Part model, mm, in its own coordinate system. A direction names the side the tool comes from. Coordinates: 2 decimals unless noted, no trailing zeros. Loops run counter-clockwise (first coordinate to the right, second up) from the corner with the lowest first, then second, coordinate; pieces in that order, holes last. Notation, with made-up numbers: (15, 34.25) - (60, 34.25) arc R35 ccw to (60, 73.25) - close; hole circle Ø5 at (41, -24). An arc over 180 degrees is marked (long way). Use a Markdown table: item, result. Add a question column.
1) Tool access for faces 4 (the face through (4.38, -8.43, 52.48)), 5 (the face through (-2.38, -10.74, 13.74)), 6 (the face through (8.11, 2.55, 139.47)), 7 (the face through (-7, 0, 122)): list every direction of +Z, -Z, +X, -X, +Y, -Y with a clear straight run to the whole face (end or side of a thin tool).
2) Probe probe 1 along Y at (x, z) = (0, 158); probe 2 along Z at (x, y) = (5, -5.5); probe 3 along Z at (x, y) = (-7.5, -4.5). List the from-to ranges inside material, lowest first. Write a range as [from, to].
3) Pull direction Z, two halves, no side cores. Call faces 1 (the face through (4.57, 7.167, 5.676)), 2 (the face through (-7, 0, 142)), 3 (the face through (2, -2, 0)): +Z half, -Z half, draft (parallel to the pull), parting line (faces both ways), or undercut.
4) Drop flat-ended pins along their axis: P1, Ø10, axis at x = 9, z = 120, coming from the +Y side; P2, Ø4, axis at x = 9.5, y = -2.5, coming from the -Z side; P3, Ø5, axis at y = -4.5, z = 23.5, coming from the -X side; P4, Ø8, axis at y = 11.5, z = 121.5, coming from the -X side. Give the stop position or say it passes through.
5) Band-saw the part on A-A (z = 104). Give the cut face in (x, y), plus the area to 3 significant figures.
from build123d import *

# Parameters (mm, degrees)
SKETCH1_R       = 8.5
EXTRUDE1_DEPTH  = 11
SKETCH2_R       = 6.5
EXTRUDE2_DEPTH  = 2
SKETCH3_R       = 11
EXTRUDE3_DEPTH  = 3
SKETCH4_R       = 9.5
EXTRUDE4_DEPTH  = 80
SKETCH5_R       = 11
EXTRUDE5_DEPTH  = 23
SKETCH6_R       = 8.25
EXTRUDE6_DEPTH  = 1
SKETCH7_R       = 8.5
EXTRUDE7_DEPTH  = 40
CHAMFER1_SIZE   = 0.5
CHAMFER2_SIZE   = 1.5
SKETCH8_R       = 2
EXTRUDE8_DEPTH  = 6
CHAMFER3_SIZE   = 2
EXTRUDE9_START  = -6
SKETCH9_R       = 2
EXTRUDE9_DEPTH  = 6
CHAMFER4_SIZE   = 2
EXTRUDE11_DEPTH = 2
LPATTERN1_COUNT = 7
LPATTERN1_PITCH = 7


with BuildPart() as part:
    # Sketch1 → Extrude1 (new body)
    with BuildSketch(Plane.XY):
        Circle(SKETCH1_R)
    extrude(amount=EXTRUDE1_DEPTH)

    # Sketch2 → Extrude2 (add)
    with BuildSketch(Plane.XY.offset(11)):
        Circle(SKETCH2_R)
    extrude(amount=EXTRUDE2_DEPTH)

    # Sketch3 → Extrude3 (add)
    with BuildSketch(Plane.XY.offset(13)):
        Circle(SKETCH3_R)
    extrude(amount=EXTRUDE3_DEPTH)

    # Sketch4 → Extrude4 (add)
    with BuildSketch(Plane.XY.offset(16)):
        Circle(SKETCH4_R)
    extrude(amount=EXTRUDE4_DEPTH)

    # Sketch5 → Extrude5 (add)
    with BuildSketch(Plane.XY.offset(96)):
        Circle(SKETCH5_R)
    extrude(amount=EXTRUDE5_DEPTH)

    # Sketch6 → Extrude6 (add)
    with BuildSketch(Plane.XY.offset(119)):
        Circle(SKETCH6_R)
    extrude(amount=EXTRUDE6_DEPTH)

    # Sketch7 → Extrude7 (add)
    with BuildSketch(Plane.XY.offset(120)):
        Circle(SKETCH7_R)
    extrude(amount=EXTRUDE7_DEPTH)

    # Chamfer1
    chamfer1_edges = [part.edges().sort_by_distance(p)[0] for p in [
        (-8.5, 0, 0),
        (-8.5, 0, 160),
    ]]
    chamfer(chamfer1_edges, length=CHAMFER1_SIZE)

    # Chamfer2
    chamfer2_edges = [part.edges().sort_by_distance(p)[0] for p in [
        (-11, 0, 96),
        (-11, 0, 16),
    ]]
    chamfer(chamfer2_edges, length=CHAMFER2_SIZE - 0.0001)  # a hair under: the kernel refuses the full size

    # Sketch8 → Extrude8 (cut)
    with BuildSketch(Plane.XY.offset(160)):
        Circle(SKETCH8_R)
    extrude(amount=-EXTRUDE8_DEPTH, mode=Mode.SUBTRACT)

    # Chamfer3
    chamfer3_edges = [part.edges().sort_by_distance(p)[0] for p in [
        (-2, 0, 154),
    ]]
    chamfer(chamfer3_edges, length=CHAMFER3_SIZE)

    # Sketch9 → Extrude9 (cut)
    with BuildSketch(Plane(origin=(0, 0, 0), x_dir=(-1, 0, 0), z_dir=(0, 0, -1)).offset(EXTRUDE9_START)):
        with Locations(Location((0, 0, 0), (0, 0, 180))):
            Circle(SKETCH9_R)
    extrude(amount=EXTRUDE9_DEPTH, mode=Mode.SUBTRACT)

    # Chamfer4
    chamfer4_edges = [part.edges().sort_by_distance(p)[0] for p in [
        (-2, 0, 6),
    ]]
    chamfer(chamfer4_edges, length=CHAMFER4_SIZE)

    # Sketch10 → Extrude11 (cut)
    with BuildSketch(Plane(origin=(-8.5, 0, 0), x_dir=(0, 0, -1), z_dir=(1, 0, 0))):
        with BuildLine():
            Line((-125, -3), (-139, -3))
            ThreePointArc((-139, -3), (-142, 0), (-139, 3))
            Line((-139, 3), (-125, 3))
            ThreePointArc((-125, 3), (-122, 0), (-125, -3))
        make_face()
    extrude(amount=EXTRUDE11_DEPTH, mode=Mode.SUBTRACT)

    # Sketch11 → Revolve1 (revolve)
    with BuildSketch(Plane(origin=(0, 0, 0), x_dir=(1, 0, 0), z_dir=(0, 1, 0))):
        Polygon((9.5, -79.265), (9.5, -74.735), (12.198447959, -75.40961199), (15.56, -76.6), (15.56, -77.4), (12.198447959, -78.59038801), align=None)
    revolve1 = revolve(axis=Axis((0, 0, 84.014072954), (0, 0, -1)))

    # LPattern1: Revolve1 ×7
    with Locations(*[(0, 0, -i * LPATTERN1_PITCH) for i in range(1, LPATTERN1_COUNT)]):
        add(revolve1)


solid = part.part
Answer block:
| question | item | result |
|---|---|---|
| 1 | face 4 | none |
| 1 | face 5 | -Z |
| 1 | face 6 | +Z |
| 1 | face 7 | -X |
| 2 | probe 1 | [-8.5, -2], [2, 8.5] |
| 2 | probe 2 | [0, 11], [13, 160] |
| 2 | probe 3 | [13, 119] |
| 3 | face 1 | draft |
| 3 | face 2 | undercut |
| 3 | face 3 | -Z half |
| 4 | P1 | y = 10.21 |
| 4 | P2 | z = 0 |
| 4 | P3 | x = -9.29 |
| 4 | P4 | x = -7.13 |
| 5 | outline | circle Ø22 at (0, 0) |
| 5 | area | 380 mm2 |
